For this review, take the finished solid that the model builds, in its own axes (mm). A direction names the side the tool comes from. Coordinates: 2 decimals unless noted, no trailing zeros. Write each loop counter-clockwise with the first axis right and the second up, starting at its lowest first coordinate (ties: lowest second). Pieces come first, ordered by that corner, then holes. Notation, with made-up numbers: (78, -23.5) -> (108, -23.5) arc R21 cw to (108, -12.5) -> close; hole circle Ø1 at (-22.75, -29.5). An arc over 180 degrees is marked (long way). One line per item, written item: value. Start each with the question number.
1) Machinability: for faces 4 (the flat face through (-41, -3, 48.786)), 5 (the flat face through (-41, -13, 50.056)), 6 (the flat face through (-8, -3, 48.786)), which of the approach directions +Z, -Z, +X, -X, +Y, -Y give a long, thin tool a straight path to every point of the face, cutting with its end or side? Answer none if there is none.
2) Add section D-D (y = -4.25). State the section outline as (x, z) points, and give its area (3 significant figures).
3) Add section C-C (y = -10.25). State the section outline as (x, z) points.
4) Add section B-B (z = 35.5). State the section outline as (x, y) points, and give its area (3 significant figures).
5) Add section A-A (x = -45.5). State the section outline as (y, z) points.
6) Mouldability with a two-part tool opening along Z and no side actions: class faces 1 (the flat face through (1, -6.35, 40)), 2 (the flat face through (25, -3, 48.786)), 3 (the flat face through (25, -13, 50.056)) as released by +Z, released by -Z, zero draft, split by the parting line, or undercut.
7) For probe 1 along X at (y, z) = (-3.5, 41.5); probe 2 along Z at (x, y) = (7.5, -2.5); probe 3 along Z at (x, y) = (43.5, -9), list the stretches that pass through material, from the lowest coordinate up. Write a range as from..to.
8) For pin 1 Ø12 at (x, z) = (15.5, 45) entering from -Y; pin 2 Ø7 at (x, y) = (-10.5, -3) entering from -Z; pin 3 Ø6.5 at (x, y) = (-28.5, -13.5) entering from -Z; pin 4 Ø8 at (x, z) = (-15.5, 40.5) entering from -Y, all flat-tipped, find the tip position at first contact; note any pin that passes through.
from build123d import *

# Parameters (mm, degrees)
F0_W     = 14.986
F0_H     = 1.27
F1_DEPTH = 1.27
F0_W_2   = 48.26
F0_H_2   = 22.86
F2_DEPTH = 6.35
F3_W     = 50.8
F3_H     = 12.7
F4_DEPTH = 0.508


# Not quite as in the source:
# - a feature names something its author has since deleted; it is built from what else it names


with BuildPart() as f1:
    # F0 (on Front) → F1 (new body)
    with BuildSketch(Plane.XZ):
        with Locations((-7.493, 49.4207651077)):
            Rectangle(F0_W, F0_H)
    extrude(amount=F1_DEPTH)

    # F0 (on Front) → F2 (join)
    with BuildSketch(Plane.XZ):
        Polygon((-14.986, 50.0557651077), (-65.786, 50.0557651077), (-65.786, 24.6557651077), (-14.986, 24.6557651077), (-14.986, 34.8157651077), (-14.986, 48.7857651077), align=None)
        with Locations((-40.386, 37.3557651077)):
            Rectangle(F0_W_2, F0_H_2, mode=Mode.SUBTRACT)
        with Locations((-7.493, 49.4207651077)):
            Rectangle(F0_W, F0_H)
        Polygon((50.8, 50.0557651077), (0, 50.0557651077), (0, 48.7857651077), (0, 34.8157651077), (0, 24.6557651077), (50.8, 24.6557651077), align=None)
        with Locations((25.4, 37.3557651077)):
            Rectangle(F0_W_2, F0_H_2, mode=Mode.SUBTRACT)
    extrude(amount=F2_DEPTH)

    # F3 (on face) → F4 (join)
    with BuildSketch(Plane.XY.offset(50.0557651077)):
        with Locations((-40.386, -12.7)):
            Rectangle(F3_W, F3_H)
        with Locations((25.4, -12.7)):
            Rectangle(F3_W, F3_H)
        Polygon((-65.786, 0), (-65.786, -6.35), (-14.986, -6.35), (0, -6.35), (50.8, -6.35), (50.8, 0), align=None)
    extrude(amount=F4_DEPTH)


solid = f1.part
Numbers:
1. face 4: +Y, -Y
1. face 5: -Z, +X, -X, -Y
1. face 6: -Z, +Y, -Y
2. outline: (-65.79, 24.66) -> (-14.99, 24.66) -> (-14.99, 48.79) -> (0, 48.79) -> (0, 24.66) -> (50.8, 24.66) -> (50.8, 50.56) -> (-65.79, 50.56) -> close; hole (-64.52, 25.93) -> (-16.26, 25.93) -> (-16.26, 48.79) -> (-64.52, 48.79) -> close; hole (1.27, 25.93) -> (49.53, 25.93) -> (49.53, 48.79) -> (1.27, 48.79) -> close
2. area: 452 mm²
3. outline: (-65.79, 50.06) -> (-14.99, 50.06) -> (-14.99, 50.56) -> (-65.79, 50.56) -> close; (0, 50.06) -> (50.8, 50.06) -> (50.8, 50.56) -> (0, 50.56) -> close
4. outline: (-65.79, -6.35) -> (-64.52, -6.35) -> (-64.52, 0) -> (-65.79, 0) -> close; (-16.26, -6.35) -> (-14.99, -6.35) -> (-14.99, 0) -> (-16.26, 0) -> close; (0, -6.35) -> (1.27, -6.35) -> (1.27, 0) -> (0, 0) -> close; (49.53, -6.35) -> (50.8, -6.35) -> (50.8, 0) -> (49.53, 0) -> close
4. area: 32.3 mm²
5. outline: (-19.05, 50.06) -> (-6.35, 50.06) -> (-6.35, 48.79) -> (0, 48.79) -> (0, 50.56) -> (-19.05, 50.56) -> close; (-6.35, 24.66) -> (0, 24.66) -> (0, 25.93) -> (-6.35, 25.93) -> close
6. face 1: zero draft
6. face 2: undercut
6. face 3: released by -Z
7. probe 1: -65.79..-64.52, -16.26..-14.99, 0..1.27, 49.53..50.8
7. probe 2: 24.66..25.93, 48.79..50.56
7. probe 3: 50.06..50.56
8. pin 1: y = -19.05
8. pin 2: z = 48.79
8. pin 3: z = 50.06
8. pin 4: y = -6.35
